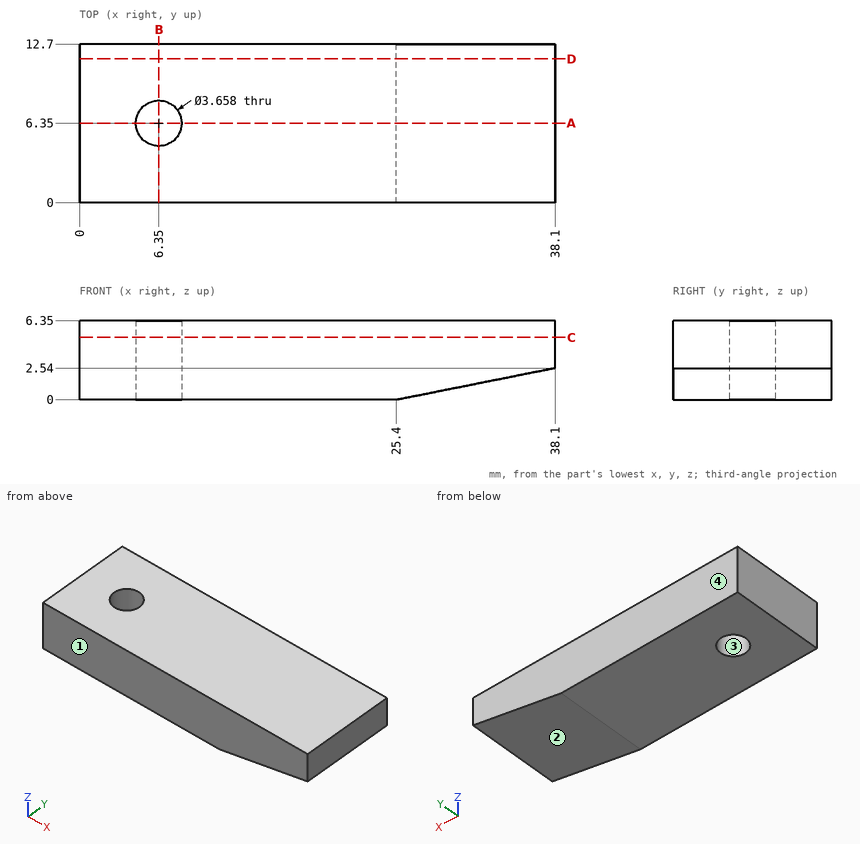
Study the drawing (mm; zero at the part's minimum x, y, z) and answer. Round coordinates to 2 decimals unless told otherwise and drop trailing zeros. Write each loop counter-clockwise with the first axis right and the second up, starting at its lowest first coordinate (ties: lowest second). Pieces come first, ordered by that corner, then holes.
1) A cutting plane is placed at A-A (y = 6.35). Give the vertices of the cut face in (x, z), plus the area to 3 significant figures.
2) The mould has two halves that part along Y. Classify the marked faces 1, 2, 3 and 4: pulls with the +Y half, pulls with the -Y half, needs draft (parallel to the pull), parting line crosses it, or undercut.
3) A cutting plane is placed at C-C (z = 5). Give the vertices of the cut face in (x, y), plus the area to 3 significant figures.
4) A cutting plane is placed at D-D (y = 11.5). Give the vertices of the cut face in (x, z).
5) A cutting plane is placed at B-B (x = 6.35). Give the vertices of the cut face in (y, z).
6) Straight lines are drawn through the part: line 1 (Y direction, x = 6.35, z = 2.5); line 2 (X direction, y = 6.25, z = 4); line 3 (Y direction, x = 6, z = 4) (1 decimal). For each, find the intervals that lie inside material, in ascending order.
Completed:
1. outline: (0, 0) - (4.52, 0) - (4.52, 6.35) - (0, 6.35) - close; (8.18, 0) - (25.4, 0) - (38.1, 2.54) - (38.1, 6.35) - (8.18, 6.35) - close
1. area: 203 mm2
2. face 1: pulls with the -Y half
2. face 2: needs draft
2. face 3: undercut
2. face 4: pulls with the +Y half
3. outline: (0, 0) - (38.1, 0) - (38.1, 12.7) - (0, 12.7) - close; hole circle Ø3.66 at (6.35, 6.35)
3. area: 473 mm2
4. outline: (0, 0) - (25.4, 0) - (38.1, 2.54) - (38.1, 6.35) - (0, 6.35) - close
5. outline: (0, 0) - (4.52, 0) - (4.52, 6.35) - (0, 6.35) - close; (8.18, 0) - (12.7, 0) - (12.7, 6.35) - (8.18, 6.35) - close
6. line 1: y = 0 to 4.52, 8.18 to 12.7
6. line 2: x = 0 to 4.52, 8.18 to 38.1
6. line 3: y = 0 to 4.6, 8.1 to 12.7
